```python
from build123d import *

# Parameters (mm, degrees)
F1_DEPTH = 950
F3_DEPTH = 950.001


with BuildPart() as f1:
    # F0 (on Top) → F1 (new body)
    with BuildSketch(Plane.XY):
        Polygon((0, -4), (0, -9.5), (136, -9.5), (136, -4), (146, -4), (146, 4), (116, 4), (110.5, 9.5), (0, 9.5), (0, 4), (12, 4), (12, -4), align=None)
    extrude(amount=F1_DEPTH)

    # F2 (on face) → F3 (cut, through all)
    with BuildSketch(Plane(origin=(0, 0, 0), x_dir=(1, 0, 0), z_dir=(0, 0, -1))):
        Polygon((107, 9.5), (107, -9.5), (110.5, -9.5), (116, -4), (146, -4), (146, 4), (136, 4), (136, 9.5), align=None)
    extrude(amount=-F3_DEPTH, mode=Mode.SUBTRACT)


solid = f1.part
```
Verification items for the finished model (mm, model axes). Give positions to 0.01 mm unless a question says otherwise; leave off trailing zeros. Loops run counter-clockwise (first coordinate to the right, second up) from the corner with the lowest first, then second, coordinate; pieces in that order, holes last.
1. Section check B-B, the plane y = -1. Enter the section's corners in (x, z).
2. Section check A-A, the plane z = 451. Enter the section's corners in (x, y).
3. Thickness scan on line 1 (Y direction, x = 10, z = 638); line 2 (X direction, y = 2.5, z = 508). Record the ranges inside material, lowest first.
4. Go/stop test with a flat-tipped pin: pin 1 Ø2.5 at (y, z) = (0, 711) entering from -X. Record where the tip stops, or that it passes through.
Geometry says:
1. outline: (12, 0) - (107, 0) - (107, 950) - (12, 950) - close
2. outline: (0, -9.5) - (107, -9.5) - (107, 9.5) - (0, 9.5) - (0, 4) - (12, 4) - (12, -4) - (0, -4) - close
3. line 1: y = -9.5 to -4, 4 to 9.5
3. line 2: x = 12 to 107
4. pin 1: stops at x = 12
